```python
from build123d import *

# Parameters (mm, degrees)
FILLET_R     = 0.5
FILLET001_R  = 0.1
SKETCH001_R  = 1.5
POCKET_DEPTH = 2


with BuildPart() as part:
    # Sketch → Revolution (revolve)
    with BuildSketch(Plane.XZ):
        Polygon((-6.5, 0), (-6.5, 1.5), (-6, 1.5), (-6, 5.75), (0, 5.75), (0, 0), align=None)
    revolve(axis=Axis((0, 0, 0), (0, 0, 1)))

    # Fillet
    fillet_edges = [part.edges().sort_by_distance(p)[0] for p in [
        (6, 0, 5.75),
    ]]
    fillet(fillet_edges, radius=FILLET_R)

    # Fillet001
    fillet001_edges = [part.edges().sort_by_distance(p)[0] for p in [
        (6.5, 0, 1.5),
        (6, 0, 1.5),
        (6.5, 0, 0),
    ]]
    fillet(fillet001_edges, radius=FILLET001_R)

    # Sketch001 (on Face9 of Fillet001) → Pocket (cut)
    with BuildSketch(Plane(origin=(0, 0, 0), x_dir=(1, 0, 0), z_dir=(0, 0, -1))):
        Circle(SKETCH001_R)
    extrude(amount=-POCKET_DEPTH, mode=Mode.SUBTRACT)


solid = part.part
```
Here's how the part is built. I have some questions about the finished solid (model axes, mm). A direction names the side the tool comes from. Coordinates: 2 decimals unless noted, no trailing zeros. Order: outer loops, then holes, each group sorted by start corner. A loop starts at its lowest first (then second) coordinate and runs counter-clockwise, first axis right, second up.
1) We'd pull the mould along X, two halves only. Please class faces 1 (the face through (6, 0, 3)), 2 (the face through (-1.5, -0.07, 0.99)), 3 (the face through (0, -2, 0)): +X half, -X half, draft (parallel to the pull), parting line (faces both ways), or undercut.
2) Will these pins go through, and if not, where does the flat tip stop? pin 1 (1 mm diameter, centred on x = -5, z = 3, fed in from +Y); pin 2 (3 mm diameter, centred on x = -3.5, z = 2, fed in from +Y); pin 3 (1.5 mm diameter, centred on x = -3.5, z = 4, fed in from -Y); pin 4 (1.5 mm diameter, centred on x = -1, y = 0, fed in from -Z).
3) Which directions (+Z, -Z, +X, -X, +Y, -Y) give clear straight access to the entire face, cutting with the end or side of a thin tool? Please do faces 4 (the face through (0, 0, 2)), 5 (the face through (0, 0, 5.75)).
4) Imagine slicing it at C-C on z = 0.9. List the corners of the cut face in (x, y) for me.
5) Imagine slicing it at A-A on y = 0. List the corners of the cut face in (x, z) for me.
6) I need wall thicknesses on line 1 (X direction, y = 0, z = 1); line 2 (Z direction, x = -4.25, y = 4.5). Which ranges of each line are inside material? Lowest first, please.
Response values:
1. face 1: parting line
1. face 2: undercut
1. face 3: draft
2. pin 1: stops at y = 3.97
2. pin 2: stops at y = 6.14
2. pin 3: stops at y = -5.33
2. pin 4: stops at z = 0
3. face 4: -Z
3. face 5: +Z, +X, -X, +Y, -Y
4. outline: circle Ø13 at (0, 0); hole circle Ø3 at (0, 0)
5. outline: (-6.5, 0.1) arc R0.1 ccw to (-6.4, 0) - (-1.5, 0) - (-1.5, 2) - (1.5, 2) - (1.5, 0) - (6.4, 0) arc R0.1 ccw to (6.5, 0.1) - (6.5, 1.4) arc R0.1 ccw to (6.4, 1.5) - (6.1, 1.5) arc R0.1 cw to (6, 1.6) - (6, 5.25) arc R0.5 ccw to (5.5, 5.75) - (-5.5, 5.75) arc R0.5 ccw to (-6, 5.25) - (-6, 1.6) arc R0.1 cw to (-6.1, 1.5) - (-6.4, 1.5) arc R0.1 ccw to (-6.5, 1.4) - close
6. line 1: x = -6.5 to -1.5, 1.5 to 6.5
6. line 2: z = 0 to 1.5
